from build123d import *

# Parameters (mm, degrees)
F0_W     = 40
F0_H     = 40
F1_DEPTH = 30
F2_R     = 4
F2_R_2   = 2
F3_DEPTH = 25
F4_DEPTH = 40
F6_DEPTH = 25


with BuildPart() as f1:
    # F0 (on Front) → F1 (new body)
    with BuildSketch(Plane.XZ):
        Rectangle(F0_W, F0_H)
    extrude(amount=F1_DEPTH)

    # F2 (on face) → F3 (join)
    with BuildSketch(Plane(origin=(0, 0, -20), x_dir=(1, 0, 0), z_dir=(0, 0, -1))):
        with Locations((0, 10)):
            Circle(F2_R)
        with Locations((0, 10)):
            Circle(F2_R_2, mode=Mode.SUBTRACT)
    extrude(amount=F3_DEPTH)

    # F4 (cut): a face of the model
    f4_faces = [f1.faces().sort_by_distance(p)[0] for p in [
        (0, -10, -20),
    ]]
    extrude(f4_faces, amount=-F4_DEPTH, mode=Mode.SUBTRACT)

    # F5 (on Right) → F6 (join, symmetric)
    with BuildSketch(Plane.YZ):
        Polygon((0, 30), (0, 0), (0, -30), (5, -30), (5, 30), align=None)
    extrude(amount=F6_DEPTH, both=True)


solid = f1.part
Part model, mm, in its own coordinate system. A direction names the side the tool comes from. Coordinates: 2 decimals unless noted, no trailing zeros. Loops run counter-clockwise (first coordinate to the right, second up) from the corner with the lowest first, then second, coordinate; pieces in that order, holes last. Notation, with made-up numbers: (-10.75, 0) -> (46.25, 0) arc R20 cw to (46.25, 4) -> close; hole circle Ø3 at (75.5, -1.5). An arc over 180 degrees is marked (long way). Use a Markdown table: item, result. Add a question column.
Item 1: Band-saw the part on A-A on x = 0. Write the cut outline in (y, z).
Item 2: Band-saw the part on D-D on z = -13. Write the cut outline in (x, y).
Item 3: Band-saw the part on C-C on z = -22. Write the cut outline in (x, y).
Item 4: Band-saw the part on B-B on y = -10. Write the cut outline in (x, z).
Item 5: Pull direction Y, two halves, no side cores. Call faces 4 (the flat face through (0, -30, 0)), 5 (the flat face through (-25, 2, 0)), 6 (the cylindrical face through (-0.521, -13.966, -32.325)), 7 (the flat face through (0, 5, 0)): +Y half, -Y half, draft (parallel to the pull), parting line (faces both ways), or undercut.
Item 6: Probe probe 1 along Y at (x, z) = (0, -33); probe 2 along X at (y, z) = (-10, -7.5); probe 3 along Y at (x, z) = (0, 10). List the from-to ranges inside material, lowest first.
Item 7: Which spindle directions (+Z, -Z, +X, -X, +Y, -Y) get a long thin tool onto all of the face, cutting with end or side? Do faces 1 (the flat face through (-20, -15, 0)), 2 (the flat face through (20, -15, 0)), 3 (the flat face through (0, -15, 20)). Say none if no direction does.
Item 8: Flat gauge pins, fed straight in: P1, Ø4.5, axis at x = 0, y = -10, coming from the +Z side; P2, Ø2, axis at x = 9.5, y = -26.5, coming from the -Z side; P3, Ø2, axis at y = -1.5, z = -12.5, coming from the +X side. Where does each tip first touch, or does it go through?
Geometry says:
| question | item | result |
|---|---|---|
| 1 | outline | (-30, -20) -> (-14, -20) -> (-14, -45) -> (-12, -45) -> (-12, 20) -> (-30, 20) -> close; (-8, -45) -> (-6, -45) -> (-6, -20) -> (0, -20) -> (0, -30) -> (5, -30) -> (5, 30) -> (0, 30) -> (0, 20) -> (-8, 20) -> close |
| 2 | outline | (-25, 0) -> (-20, 0) -> (-20, -30) -> (20, -30) -> (20, 0) -> (25, 0) -> (25, 5) -> (-25, 5) -> close; hole circle Ø4 at (0, -10) |
| 3 | outline | (-25, 0) -> (25, 0) -> (25, 5) -> (-25, 5) -> close; circle Ø8 at (0, -10); hole circle Ø4 at (0, -10) |
| 4 | outline | (-20, -20) -> (-4, -20) -> (-4, -45) -> (-2, -45) -> (-2, 20) -> (-20, 20) -> close; (2, -45) -> (4, -45) -> (4, -20) -> (20, -20) -> (20, 20) -> (2, 20) -> close |
| 5 | face 4 | -Y half |
| 5 | face 5 | draft |
| 5 | face 6 | undercut |
| 5 | face 7 | +Y half |
| 6 | probe 1 | -14 to -12, -8 to -6 |
| 6 | probe 2 | -20 to -2, 2 to 20 |
| 6 | probe 3 | -30 to -12, -8 to 5 |
| 7 | face 1 | +Z, -Z, -X, -Y |
| 7 | face 2 | +Z, -Z, +X, -Y |
| 7 | face 3 | +Z, +X, -X, -Y |
| 8 | P1 | z = 20 |
| 8 | P2 | z = -20 |
| 8 | P3 | x = 20 |
